Check sheet for the modelled part. Datum: model origin and axes. Units: mm. Coordinates: 2 decimals unless noted, no trailing zeros. Loops run counter-clockwise (first coordinate to the right, second up) from the corner with the lowest first, then second, coordinate; pieces in that order, holes last.
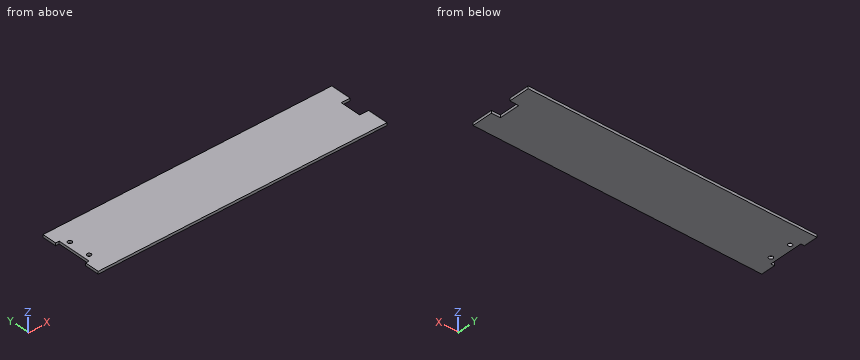
Autodesk Inventor part; units mm, degrees
ref_plane "YZ Plane" through (0, 0, 0) normal (1, 0, 0) x (0, 1, 0)
ref_plane "XZ Plane" through (0, 0, 0) normal (0, 1, 0) x (-1, 0, 0)
ref_plane "XY Plane" through (0, 0, 0) normal (0, 0, 1) x (1, 0, 0)
sketch "Sketch1" plane through (0, 0, 0) normal (0, 0, 1) x (1, 0, 0)
  line L0 (0, 0) -> (352.552, 0)
  line L1 (352.552, 0) -> (352.552, 76.2)
  line L2 (352.552, 76.2) -> (0, 76.2)
  line L3 (0, 76.2) -> (0, 0)
  circle A0 centre (10.795, 51.308) radius 2.54
  circle A1 centre (10.795, 24.892) radius 2.54
  line L4 (102.1122, 0) -> (121.213, 0)
  line L5 (102.1122, 0) -> (83.0114, 0)
  line L6 (0, 76.2) -> (10.795, 76.2)
  line L7 (0, 63.0428) -> (0, 24.8412)
  line L8 (0, 76.2) -> (10.795, 76.2)
  line L9 (3.81, 38.1) -> (3.81, 58.1025)
  line L10 (3.81, 58.1025) -> (0, 58.1025)
  line L11 (3.81, 38.1) -> (3.81, 18.0975)
  line L12 (3.81, 18.0975) -> (0, 18.0975)
  line L13 (3.81, 38.1) -> (3.81, 58.1025)
  line L14 (0, 58.1025) -> (3.81, 58.1025)
  line L15 (3.81, 58.1025) -> (3.81, 18.0975)
  line L16 (3.81, 18.0975) -> (0, 18.0975)
  line L17 (0, 18.0975) -> (0, 58.1025)
  dimension "d0" = 352.552
  dimension "d1" = 76.2
  dimension "d15" = 20.0025
extrude "Extrusion1" add sketch "Sketch1" along normal blind 3.175
sketch "Sketch2" plane through (0, 0, 3.175) normal (0, 0, 1) x (1, 0, 0)
  line L0 (352.552, 76.2) -> (0, 76.2)
  line L1 (352.552, 0) -> (352.552, 76.2)
  line L2 (352.552, 50.8) -> (339.852, 50.8)
  line L3 (339.852, 50.8) -> (339.852, 25.4)
  line L4 (339.852, 25.4) -> (352.552, 25.4)
  line L5 (352.552, 25.4) -> (352.552, 50.8)
  point P0 (0, 0)
  dimension "d6" = 25.4
  dimension "d7" = 12.7
  dimension "d8" = 25.4
extrude "Extrusion2" cut sketch "Sketch2" against normal blind 25.4
sketch "Sketch3" plane through (0, 0, 3.175) normal (0, 0, 1) x (1, 0, 0)
  point P0 (0, 0)
sketch "Sketch4" plane through (0, 0, 3.175) normal (0, 0, 1) x (1, 0, 0)
  point P0 (0, 0)
sketch "Sketch5" plane through (0, 0, 3.175) normal (0, 0, 1) x (1, 0, 0)
  circle A0 centre (10.795, 51.308) radius 2.54
  circle A1 centre (10.795, 24.892) radius 2.54
  line L0 (0, 76.2) -> (0, 0)
  line L1 (0, 38.1) -> (0, 58.7375)
  line L2 (0, 58.7375) -> (4.3688, 58.7375)
  line L3 (4.3688, 58.7375) -> (4.3688, 17.4625)
  line L4 (4.3688, 17.4625) -> (0, 17.4625)
  line L5 (0, 17.4625) -> (0, 38.1)
  point P0 (0, 17.4625)
  dimension "d16" = 20.6375
  dimension "d17" = 4.3688
extrude "Extrusion3" cut sketch "Sketch5" against normal blind 25.4 contours L2 L3 L4 L0
sketch "Sketch6" plane through (0, 0, 3.175) normal (0, 0, 1) x (1, 0, 0)
  line L0 (352.552, 50.8) -> (352.552, 76.2)
  line L1 (0, 0) -> (352.552, 0)
  line L2 (352.552, 76.2) -> (350.647, 76.2)
  line L3 (350.647, 76.2) -> (350.647, 0)
  line L4 (350.647, 0) -> (352.552, 0)
  line L5 (352.552, 0) -> (352.552, 76.2)
  point P0 (352.552, 0)
  dimension "d21" = 1.905
extrude "Extrusion4" cut sketch "Sketch6" against normal blind 25.4
properties part number "220310 Back Cover"
(1) Section check B-B, the plane y = 33.5. Enter the section's corners in (x, z) (3 decimals).
(2) Scan lines: line 1 along X through (y, z) = (50, 0.35); line 2 along X through (y, z) = (41, 3); line 3 along X through (y, z) = (17.5, 0.65). Record each from-to range of solid material in increasing order.
(3) Section check A-A, the plane z = 2. Enter the section's corners in (x, y) (1 decimal).
(4) Gauge pin test, flat ends, axial feed: P1, Ø1, axis at y = 33, z = 2, coming from the -X side; P2, Ø3, axis at x = 10.795, y = 51.308, coming from the -Z side. Record the tip position at first contact, or that the pin passes through.
Determined:
1. outline: (4.369, 0) - (339.852, 0) - (339.852, 3.175) - (4.369, 3.175) - close
2. line 1: x = 4.37 to 8.62, 12.97 to 339.85
2. line 2: x = 4.37 to 339.85
2. line 3: x = 4.37 to 350.65
3. outline: (0, 0) - (350.6, 0) - (350.6, 25.4) - (339.9, 25.4) - (339.9, 50.8) - (350.6, 50.8) - (350.6, 76.2) - (0, 76.2) - (0, 58.7) - (4.4, 58.7) - (4.4, 17.5) - (0, 17.5) - close; hole circle Ø5.1 at (10.8, 24.9); hole circle Ø5.1 at (10.8, 51.3)
4. P1: stops at x = 4.37
4. P2: passes through
